Can you work these out from the model? Positions are in its coordinate system, mm. A direction names the side the tool comes from. Give positions to 0.01 mm unless a question says otherwise; leave off trailing zeros. Write each loop counter-clockwise with the first axis right and the second up, starting at its lowest first coordinate (ties: lowest second). Pieces come first, ordered by that corner, then holes.
1. Suppose I cut it at D-D (y = -7). Please give me the cut outline in (x, z), and give its area (4 significant figures).
2. Suppose I cut it at A-A (z = 1.1). Please give me the cut outline in (x, y), and give its area (3 significant figures).
3. Suppose I cut it at B-B (y = 0.75). Please give me the cut outline in (x, z).
4. Thinking about a two-plate mould opening in Y: for faces 4 (the flat face through (3, 11, 2)), 5 (the flat face through (-4.5, 2, 2.7)), 6 (the flat face through (5, 0, 1)), which applies, pulls with the +Y half, pulls with the -Y half, needs draft (parallel to the pull), parting line crosses it, or undercut?
5. If I drill on probe 1 along X at (y, z) = (-10, 3.4); probe 2 along Y at (x, z) = (2.5, 2.85); probe 3 along X at (y, z) = (2.5, 1.8), over which ranges is the centre line in solid material (lowest first)?
6. Suppose I cut it at C-C (x = 4.25). Please give me the cut outline in (y, z), and give its area (3 significant figures).
7. I'm going to push flat-ended pins straight in: pin 1 (0.8 mm diameter, centred on x = 0, z = 2.5, fed in from -Y); pin 2 (0.8 mm diameter, centred on x = -0.5, y = -9, fed in from -Z); pin 3 (2 mm diameter, centred on x = 1, z = 3, fed in from -Y); pin 4 (1.2 mm diameter, centred on x = -0.5, z = 2.5, fed in from +Y). Where does each tip first touch, or does it pass through?
8. On a 3-axis mill with a long thin cutter (end or side, diameter ignored), from which of +Z, -Z, +X, -X, +Y, -Y can I reach the whole of each face in a straight line? I mean faces 1 (the flat face through (-4.5, -2, 2.7)), 2 (the flat face through (0, -9.4, 1.5)), 3 (the flat face through (0, -8.9, 3)). Say none if no direction works.
```python
from build123d import *

# Parameters (mm, degrees)
SKETCH1_W           = 10
SKETCH1_H           = 22
BOSS_EXTRUDE1_DEPTH = 4
SKETCH2_W           = 3.5
SKETCH2_H           = 22
SLOT_DEPTH          = 1.5
SKETCH3_W           = 3.5
SKETCH3_H           = 1.1
CUT_EXTRUDE2_DEPTH  = 2.5
SKETCH4_W           = 8
SKETCH4_H           = 17.8
CUT_EXTRUDE3_DEPTH  = 2.5
CUT_EXTRUDE4_REACH  = 17.395
SKETCH6_W           = 2.5
SKETCH6_H           = 4


with BuildPart() as part:
    # Sketch1 → Boss-Extrude1 (new body)
    with BuildSketch(Plane.XY):
        Rectangle(SKETCH1_W, SKETCH1_H)
    extrude(amount=BOSS_EXTRUDE1_DEPTH)

    # Sketch2 → slot (cut)
    with BuildSketch(Plane(origin=(0, 0, 0), x_dir=(-1, 0, 0), z_dir=(0, 0, -1))):
        Rectangle(SKETCH2_W, SKETCH2_H)
    extrude(amount=-SLOT_DEPTH, mode=Mode.SUBTRACT)

    # Sketch3 → Cut-Extrude2 (cut)
    with BuildSketch(Plane(origin=(0, 0, 1.5), x_dir=(-1, 0, 0), z_dir=(0, 0, -1))):
        with Locations((0, 10.45)):
            Rectangle(SKETCH3_W, SKETCH3_H)
        with Locations((0, -10.45)):
            Rectangle(SKETCH3_W, SKETCH3_H)
    extrude(amount=-CUT_EXTRUDE2_DEPTH, mode=Mode.SUBTRACT)

    # Sketch4 → Cut-Extrude3 (cut)
    with BuildSketch(Plane.XY.offset(4)):
        Rectangle(SKETCH4_W, SKETCH4_H)
    extrude(amount=-CUT_EXTRUDE3_DEPTH, mode=Mode.SUBTRACT)

    # Cut-Extrude4: up to this face of the body (flat: up to its plane)
    cut_extrude4_end = Plane(part.part.faces().sort_by_distance((5, 0, 2))[0])
    # Sketch6 → Cut-Extrude4 (cut, up to the picked face)
    with BuildSketch(Plane.ZY.offset(5), mode=Mode.PRIVATE) as cut_extrude4_sk1:
        with Locations((2.75, 0)):
            Rectangle(SKETCH6_W, SKETCH6_H)
    cut_extrude4_tool1 = split(extrude(cut_extrude4_sk1.sketch, amount=-CUT_EXTRUDE4_REACH, mode=Mode.PRIVATE), bisect_by=cut_extrude4_end, keep=Keep.BOTH, mode=Mode.PRIVATE)
    add(cut_extrude4_tool1.solids().sort_by(Axis((-5, 0, 2.75), (1, 0, 0)))[0], mode=Mode.SUBTRACT)


solid = part.part
```
Checks:
1. outline: (-5, 0) - (-1.75, 0) - (-1.75, 1.5) - (-4, 1.5) - (-4, 4) - (-5, 4) - close; (1.75, 0) - (5, 0) - (5, 4) - (4, 4) - (4, 1.5) - (1.75, 1.5) - close
1. area: 14.75 mm2
2. outline: (-5, -11) - (-1.75, -11) - (-1.75, 11) - (-5, 11) - close; (1.75, -11) - (5, -11) - (5, 11) - (1.75, 11) - close
2. area: 143 mm2
3. outline: (-5, 0) - (-1.75, 0) - (-1.75, 1.5) - (-5, 1.5) - close; (1.75, 0) - (5, 0) - (5, 1.5) - (1.75, 1.5) - close
4. face 4: pulls with the +Y half
4. face 5: undercut
4. face 6: needs draft
5. probe 1: x = -5 to -1.75, 1.75 to 5
5. probe 2: y = -11 to -8.9, 8.9 to 11
5. probe 3: x = -5 to -4, 4 to 5
6. outline: (-11, 0) - (11, 0) - (11, 4) - (2, 4) - (2, 1.5) - (-2, 1.5) - (-2, 4) - (-11, 4) - close
6. area: 78.0 mm2
7. pin 1: stops at y = -9.9
7. pin 2: stops at z = 1.5
7. pin 3: stops at y = -11
7. pin 4: stops at y = 9.9
8. face 1: +Z, +X, -X
8. face 2: -Z, +Y, -Y
8. face 3: +Z
